from build123d import *

# Parameters (mm, degrees)
SKETCH1_W           = 24
SKETCH1_H           = 8
BOSS_EXTRUDE1_DEPTH = 6
SKETCH2_W           = 24
SKETCH2_H           = 12
BOSS_EXTRUDE2_DEPTH = 1.5
SKETCH3_R           = 2.5
SKETCH3_W           = 6
SKETCH3_H           = 4
CUT_EXTRUDE1_DEPTH  = 16.370426149
CHAMFER1_SIZE       = 0.25


with BuildPart() as part:
    # Sketch1 → Boss-Extrude1 (new body)
    with BuildSketch(Plane.XY):
        Rectangle(SKETCH1_W, SKETCH1_H)
    extrude(amount=-BOSS_EXTRUDE1_DEPTH)

    # Sketch2 → Boss-Extrude2 (add)
    with BuildSketch(Plane(origin=(0, 0, -6), x_dir=(-1, 0, 0), z_dir=(0, 0, -1))):
        Rectangle(SKETCH2_W, SKETCH2_H)
    extrude(amount=BOSS_EXTRUDE2_DEPTH)

    # Sketch3 → Cut-Extrude1 (cut, through all)
    with BuildSketch(Plane.XY):
        Circle(SKETCH3_R)
        with Locations((-7, 0)):
            Rectangle(SKETCH3_W, SKETCH3_H)
        with Locations((7, 0)):
            Rectangle(SKETCH3_W, SKETCH3_H)
    extrude(amount=-CUT_EXTRUDE1_DEPTH, mode=Mode.SUBTRACT)

    # Chamfer1
    chamfer1_edges = [part.edges().sort_by_distance(p)[0] for p in [
        (12, 5, -6),
        (12, -5, -6),
        (0, -6, -6),
        (12, -6, -6.75),
        (-12, -5, -6),
        (0, 4, -6),
        (-12, 5, -6),
        (0, 6, -6),
        (12, 0, -7.5),
        (0, -6, -7.5),
        (-12, 0, -7.5),
        (0, 6, -7.5),
        (0, 4, 0),
        (12, 0, 0),
        (0, -4, 0),
        (-12, 0, 0),
        (-12, 4, -3),
        (12, 4, -3),
        (12, -4, -3),
        (-12, -4, -3),
        (0, -4, -6),
    ]]
    chamfer(chamfer1_edges, length=CHAMFER1_SIZE)


solid = part.part
Verification items for the finished model (mm, model axes). A direction names the side the tool comes from. Round coordinates to 2 decimals unless told otherwise and drop trailing zeros. Loops run counter-clockwise (first coordinate to the right, second up) from the corner with the lowest first, then second, coordinate; pieces in that order, holes last. Notation, with made-up numbers: (61, -39.5) - (117, -39.5) arc R18 cw to (117, -32.5) - close; hole circle Ø4 at (6.25, 9). An arc over 180 degrees is marked (long way). Answer in a Markdown table with one row per item. Add a question column.
Q1. Section check D-D on y = 4.5. Enter the section's corners in (x, z), plus the area to 3 significant figures.
Q2. Section check A-A on x = 4.25. Enter the section's corners in (y, z).
Q3. Tool access check on faces 1 (the face through (0, -5, -6)), 2 (the face through (-10, 0, -4)), 3 (the face through (0, 3, 0)), 4 (the face through (0, 4, -3)). Record the directions out of +Z, -Z, +X, -X, +Y, -Y that give a thin tool (end or side, any length) a straight path to the whole face; none if there is none.
Q4. Material ranges on line 1 (X direction, y = 1.5, z = -4); line 2 (Y direction, x = 0, z = -4); line 3 (Y direction, x = -9.75, z = -5.5), recorded low to high.
Q5. Section check B-B on z = -4.25. Enter the section's corners in (x, y), plus the area to 3 significant figures.
Q6. Gauge pin test, flat ends, axial feed: pin 1 (3 mm diameter, centred on x = -8, z = -4, fed in from +Y); pin 2 (1 mm diameter, centred on x = -6, z = -5, fed in from -Y); pin 3 (4 mm diameter, centred on x = 0, y = 0, fed in from +Z); pin 4 (0.8 mm diameter, centred on x = -0.5, y = 5, fed in from +Z). Record the tip position at first contact, or that the pin passes through.
Q7. Section check C-C on y = 0. Enter the section's corners in (x, z).
Found:
| question | item | result |
|---|---|---|
| 1 | outline | (-12, -7.25) - (-11.75, -7.5) - (11.75, -7.5) - (12, -7.25) - (12, -6.25) - (11.75, -6) - (-11.75, -6) - (-12, -6.25) - close |
| 1 | area | 35.9 mm² |
| 2 | outline | (-6, -7.25) - (-5.75, -7.5) - (-2, -7.5) - (-2, 0) - (-3.75, 0) - (-4, -0.25) - (-4, -5.75) - (-4.25, -6) - (-5.75, -6) - (-6, -6.25) - close; (2, -7.5) - (5.75, -7.5) - (6, -7.25) - (6, -6.25) - (5.75, -6) - (4.25, -6) - (4, -5.75) - (4, -0.25) - (3.75, 0) - (2, 0) - close |
| 3 | face 1 | +Z, +X, -X, -Y |
| 3 | face 2 | +Z, -Z |
| 3 | face 3 | +Z, +X, -X, +Y, -Y |
| 3 | face 4 | +Z, +X, -X, +Y |
| 4 | line 1 | x = -12 to -10, -4 to -2, 2 to 4, 10 to 12 |
| 4 | line 2 | y = -4 to -2.5, 2.5 to 4 |
| 4 | line 3 | y = -4 to -2, 2 to 4 |
| 5 | outline | (-12, -3.75) - (-11.75, -4) - (11.75, -4) - (12, -3.75) - (12, 3.75) - (11.75, 4) - (-11.75, 4) - (-12, 3.75) - close; hole (-10, -2) - (-4, -2) - (-4, 2) - (-10, 2) - close; hole circle Ø5 at (0, 0); hole (4, -2) - (10, -2) - (10, 2) - (4, 2) - close |
| 5 | area | 124 mm² |
| 6 | pin 1 | stops at y = 4 |
| 6 | pin 2 | stops at y = -4 |
| 6 | pin 3 | passes through |
| 6 | pin 4 | stops at z = -6 |
| 7 | outline | (-12, -7.25) - (-11.75, -7.5) - (-10, -7.5) - (-10, 0) - (-11.75, 0) - (-12, -0.25) - close; (-4, -7.5) - (-2.5, -7.5) - (-2.5, 0) - (-4, 0) - close; (2.5, -7.5) - (4, -7.5) - (4, 0) - (2.5, 0) - close; (10, -7.5) - (11.75, -7.5) - (12, -7.25) - (12, -0.25) - (11.75, 0) - (10, 0) - close |
